The figure shows three views and two pictorial views of one solid part (mm, origin at its lowest corner). Answer the questions. Round coordinates to 2 decimals unless told otherwise and drop trailing zeros. Write each loop counter-clockwise with the first axis right and the second up, starting at its lowest first coordinate (ties: lowest second). Pieces come first, ordered by that corner, then holes. Notation, with made-up numbers: (-27, 49.25) - (3, 49.25) arc R28 ccw to (3, 83.25) - close; hole circle Ø9 at (-20, 71.5). An arc over 180 degrees is marked (long way). Answer as CSV lines item,"result". Start each with the question number.
Item 1: A cutting plane is placed at C-C on x = 45. Determine the outline of the cut face in (y, z).
Item 2: A cutting plane is placed at A-A on x = 8. Determine the outline of the cut face in (y, z).
Item 3: A cutting plane is placed at B-B on y = 15. Determine the outline of the cut face in (x, z).
Item 4: A flat-ended cylindrical pin translates along its axis: pin 1 (4 mm diameter, centred on x = 40.5, y = 11, fed in from +Z). Find the tip coordinate at first contact, or state that the pin passes through.
Item 5: Straight lines are drawn through the part: line 1 along X through (y, z) = (15, 2); line 2 along Y through (x, z) = (8, 2.1); line 3 along X through (y, z) = (14, 0.3). For each, find the intervals that lie inside material, in ascending order. Write a range as [from, to].
Item 6: A cutting plane is placed at D-D on y = 22.5. Determine the outline of the cut face in (x, z).
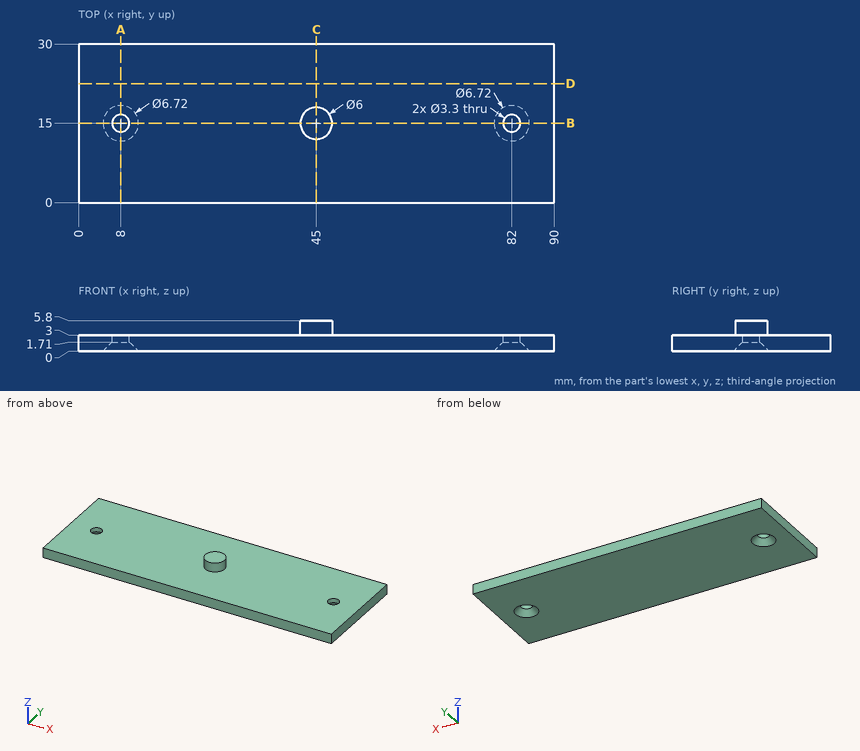
Geometry says:
1,outline,"(0, 0) - (30, 0) - (30, 3) - (18, 3) - (18, 5.8) - (12, 5.8) - (12, 3) - (0, 3) - close"
2,outline,"(0, 0) - (11.64, 0) - (13.35, 1.71) - (13.35, 3) - (0, 3) - close; (16.65, 1.71) - (18.36, 0) - (30, 0) - (30, 3) - (16.65, 3) - close"
3,outline,"(0, 0) - (4.64, 0) - (6.35, 1.71) - (6.35, 3) - (0, 3) - close; (9.65, 1.71) - (11.36, 0) - (78.64, 0) - (80.35, 1.71) - (80.35, 3) - (48, 3) - (48, 5.8) - (42, 5.8) - (42, 3) - (9.65, 3) - close; (83.65, 1.71) - (85.36, 0) - (90, 0) - (90, 3) - (83.65, 3) - close"
4,pin 1,"stops at z = 3"
5,line 1,"x = [0, 6.35], [9.65, 80.35], [83.65, 90]"
5,line 2,"y = [0, 13.35], [16.65, 30]"
5,line 3,"x = [0, 5.11], [10.89, 79.11], [84.89, 90]"
6,outline,"(0, 0) - (90, 0) - (90, 3) - (0, 3) - close"
